```python
from build123d import *

# Parameters (mm, degrees)
SKETCH1_W                      = 27
SKETCH1_H                      = 35
SKETCH1_R                      = 1.113712744
SKETCH1_R_2                    = 1.000106258
SKETCH1_R_3                    = 1.174626552
SKETCH1_R_4                    = 1.19920455
SKETCH1_W_2                    = 8.5
SKETCH1_H_2                    = 2.12
BOSS_EXTRUDE1_DEPTH            = 2
SKETCH3_R                      = 2
BOSS_EXTRUDE2_DEPTH            = 2
M2_CLEARANCE_HOLE1_D           = 2.4
LPATTERN1_COUNT                = 2
LPATTERN1_PITCH                = 18
LPATTERN1_COUNT_DIR2           = 2
LPATTERN1_PITCH_DIR2           = 21.5
SKETCH6_W                      = 27
SKETCH6_H                      = 35
SKETCH6_W_2                    = 24
SKETCH6_H_2                    = 32
BOSS_EXTRUDE4_DEPTH            = 8.32
CUT_EXTRUDE1_REACH             = 41.261
SKETCH7_W                      = 8.5
SKETCH7_H                      = 5.57
CUT_EXTRUDE1_DIRECTION_2_DEPTH = 40.260756636
BOSS_EXTRUDE5_START            = -4
BOSS_EXTRUDE5_OUTLINE_R        = 1.2
BOSS_EXTRUDE5_DEPTH            = 2
M2_CLEARANCE_HOLE2_D           = 2.4
FILLET1_R                      = 2


with BuildPart() as part:
    # Sketch1 → Boss-Extrude1 (new body)
    # profile 1 of 8: a face of its own
    with BuildSketch(Plane(origin=(0, 0, 0), x_dir=(1, 0, 0), z_dir=(0, 1, 0))):
        with Locations((0.988085162, -0.939800033)):
            Rectangle(SKETCH1_W, SKETCH1_H)
        Polygon((-10.011914838, -15.939800033), (-10.011914838, 14.060199967), (11.988085162, 14.060199967), (11.988085162, -15.939800033), (5.238085162, -15.939800033), (5.238085162, -18.059800033), (-3.261914838, -18.059800033), (-3.261914838, -15.939800033), align=None, mode=Mode.SUBTRACT)
    # profile 2 of 8: a face of its own
    with BuildSketch(Plane(origin=(0, 0, 0), x_dir=(1, 0, 0), z_dir=(0, 1, 0))):
        Polygon((11.988085162, 14.060199967), (-10.011914838, 14.060199967), (-10.011914838, -15.939800033), (-3.261914838, -15.939800033), (-3.261914838, -13.819800033), (5.238085162, -13.819800033), (5.238085162, -15.939800033), (11.988085162, -15.939800033), align=None)
        with Locations((-8.011914838, -13.939800033)):
            Circle(SKETCH1_R, mode=Mode.SUBTRACT)
        with Locations((7.931487186, -14.291814947)):
            Circle(SKETCH1_R_2, mode=Mode.SUBTRACT)
        with Locations((-8.011914838, 7.560199967)):
            Circle(SKETCH1_R_3, mode=Mode.SUBTRACT)
        with Locations((9.988085162, 7.560199967)):
            Circle(SKETCH1_R_4, mode=Mode.SUBTRACT)
    # profile 3 of 8: a face of its own
    with BuildSketch(Plane(origin=(0, 0, 0), x_dir=(1, 0, 0), z_dir=(0, 1, 0))):
        with Locations((-8.011914838, 7.560199967)):
            Circle(SKETCH1_R_3)
    # profile 4 of 8: a face of its own
    with BuildSketch(Plane(origin=(0, 0, 0), x_dir=(1, 0, 0), z_dir=(0, 1, 0))):
        with Locations((9.988085162, 7.560199967)):
            Circle(SKETCH1_R_4)
    # profile 5 of 8: a face of its own
    with BuildSketch(Plane(origin=(0, 0, 0), x_dir=(1, 0, 0), z_dir=(0, 1, 0))):
        with Locations((7.931487186, -14.291814947)):
            Circle(SKETCH1_R_2)
    # profile 6 of 8: a face of its own
    with BuildSketch(Plane(origin=(0, 0, 0), x_dir=(1, 0, 0), z_dir=(0, 1, 0))):
        with Locations((0.988085162, -16.999800033)):
            Rectangle(SKETCH1_W_2, SKETCH1_H_2)
    # profile 7 of 8: a face of its own
    with BuildSketch(Plane(origin=(0, 0, 0), x_dir=(1, 0, 0), z_dir=(0, 1, 0))):
        with Locations((0.988085162, -14.879800033)):
            Rectangle(SKETCH1_W_2, SKETCH1_H_2)
    # profile 8 of 8: a face of its own
    with BuildSketch(Plane(origin=(0, 0, 0), x_dir=(1, 0, 0), z_dir=(0, 1, 0))):
        with Locations((-8.011914838, -13.939800033)):
            Circle(SKETCH1_R)
    extrude(amount=BOSS_EXTRUDE1_DEPTH)

    # Sketch3 → Boss-Extrude2 (add)
    with BuildSketch(Plane(origin=(0, 2, 0), x_dir=(1, 0, 0), z_dir=(0, 1, 0))):
        with Locations(Location((-8.011914838, 7.560199967, 0), (0, 0, 270))):
            Circle(SKETCH3_R)
    boss_extrude2 = extrude(amount=BOSS_EXTRUDE2_DEPTH)

    # M2 Clearance Hole1 (through all)
    with Locations(Plane(origin=(0, 4, 0), x_dir=(1, 0, 0), z_dir=(0, 1, 0))):
        with Locations((-8.011914838, 7.560199967)):
            m2_clearance_hole1 = Hole(M2_CLEARANCE_HOLE1_D / 2)

    # LPattern1: Boss-Extrude2, M2 Clearance Hole1 2 × 2
    with Locations(*[(i * LPATTERN1_PITCH, 0, j * LPATTERN1_PITCH_DIR2) for i in range(LPATTERN1_COUNT) for j in range(LPATTERN1_COUNT_DIR2) if (i, j) != (0, 0)]):
        add(boss_extrude2)
        add(m2_clearance_hole1, mode=Mode.SUBTRACT)

    # Sketch6 → Boss-Extrude4 (add)
    with BuildSketch(Plane(origin=(0, 2, 0), x_dir=(1, 0, 0), z_dir=(0, 1, 0))):
        with Locations((0.988085162, -0.939800033)):
            Rectangle(SKETCH6_W, SKETCH6_H)
        with Locations((0.988085162, -0.939800033)):
            Rectangle(SKETCH6_W_2, SKETCH6_H_2, mode=Mode.SUBTRACT)
    extrude(amount=BOSS_EXTRUDE4_DEPTH)

    # Sketch7 → Cut-Extrude1 (cut, up to next)
    with BuildSketch(Plane.XY.offset(18.439800033), mode=Mode.PRIVATE) as cut_extrude1_sk1:
        with Locations((0.988085162, 7.535)):
            Rectangle(SKETCH7_W, SKETCH7_H)
    cut_extrude1_tool1 = extrude(cut_extrude1_sk1.sketch, amount=-CUT_EXTRUDE1_REACH, mode=Mode.PRIVATE) & part.part
    add(cut_extrude1_tool1.solids().sort_by_distance((0.988085, 7.535, 18.4398))[0], mode=Mode.SUBTRACT)

    # Sketch7 → Cut-Extrude1 direction 2 (cut)
    with BuildSketch(Plane.XY.offset(18.439800033)):
        with Locations((0.988085162, 7.535)):
            Rectangle(SKETCH7_W, SKETCH7_H)
    extrude(amount=CUT_EXTRUDE1_DIRECTION_2_DEPTH, mode=Mode.SUBTRACT)

    # Boss-Extrude5: read off the stored shape, not the designer's step
    # Boss-Extrude5 outline → Boss-Extrude5 (add)
    with BuildSketch(Plane(origin=(0, 12.32, 0), x_dir=(1, 0, 0), z_dir=(0, 1, 0)).offset(BOSS_EXTRUDE5_START)):
        Polygon((-5.169409796, -23.439799853), (-5.169409796, -18.439799853), (-12.511914838, -18.439800033), (-12.511914838, 16.560199967), (14.488085162, 16.560199967), (14.488085162, -18.439800033), (7.002600417, -18.439800033), (7.002600417, -23.439799853), (19.488084722, -23.439799853), (19.488084722, 21.560200147), (-17.511915278, 21.560200147), (-17.511915278, -23.439799853), align=None)
        with Locations((-15.011915278, -20.939799853)):
            Circle(BOSS_EXTRUDE5_OUTLINE_R, mode=Mode.SUBTRACT)
        with Locations((16.988084722, -20.939799853)):
            Circle(BOSS_EXTRUDE5_OUTLINE_R, mode=Mode.SUBTRACT)
        with Locations((-15.011915278, 0)):
            Circle(BOSS_EXTRUDE5_OUTLINE_R, mode=Mode.SUBTRACT)
        with Locations((-15.011915278, 19.060200147)):
            Circle(BOSS_EXTRUDE5_OUTLINE_R, mode=Mode.SUBTRACT)
        with Locations((16.988084722, -0.939799853)):
            Circle(BOSS_EXTRUDE5_OUTLINE_R, mode=Mode.SUBTRACT)
        with Locations((16.988084722, 19.060200147)):
            Circle(BOSS_EXTRUDE5_OUTLINE_R, mode=Mode.SUBTRACT)
    extrude(amount=BOSS_EXTRUDE5_DEPTH)

    # M2 Clearance Hole2 (through all)
    with Locations(Plane(origin=(0, 10.32, 0), x_dir=(1, 0, 0), z_dir=(0, 1, 0))):
        with Locations((-15.011915278, 19.060200147), (-15.011915278, 0), (-15.011915278, -20.939799853), (16.988084722, -20.939799853), (16.988084722, -0.939799853), (16.988084722, 19.060200147)):
            Hole(M2_CLEARANCE_HOLE2_D / 2)

    # Fillet1
    # the kernel refuses this fillet: 2 mm, written as the material it adds along each edge
    with BuildSketch(Plane(origin=(7.002600417, 8.32, 18.439800033), x_dir=(0, 0, 1), z_dir=(0, 1, 0))) as fillet1_piece_1:
        with BuildLine():
            CenterArc((1.98608835, -2), FILLET1_R, 90, 83.23817367)
            Line((0, -1.764515255), (-0.039721767, -1.75980556))
            ThreePointArc((-0.039721767, -1.75980556), (-0.04, -0.882257627), (-0.04, 0))
            Line((-0.04, 0), (0, 0.04))
            Line((0, 0.04), (1.98608835, 0.04))
            Line((1.98608835, 0.04), (1.98608835, 0))
        make_face()
    extrude(amount=2)
    # the kernel refuses this fillet: 2 mm, written as the material it adds along each edge
    with BuildSketch(Plane(origin=(-5.169409796, 8.32, 18.439799853), x_dir=(0, 0, 1), z_dir=(0, 1, 0))) as fillet1_2_piece_1:
        with BuildLine():
            CenterArc((1.997859739, 2), FILLET1_R, 182.651020031, 87.348979969)
            Line((1.8e-07, 1.907494958), (-0.039957011, 1.905644857))
            ThreePointArc((-0.039957011, 1.905644857), (-0.03999982, 0.953747479), (-0.04, 0))
            Line((-0.04, 0), (0, -0.04))
            Line((0, -0.04), (1.997859739, -0.04))
            Line((1.997859739, -0.04), (1.997859739, 0))
        make_face()
    extrude(amount=2)
    # the kernel refuses this fillet: 2 mm, written as the material it takes off along each edge
    with BuildSketch(Plane(origin=(-5.169409796, 3.32, 23.439799853), x_dir=(0, 0, -1), z_dir=(0, 1, 0))) as fillet1_3_piece_1:
        with BuildLine():
            CenterArc((FILLET1_R, FILLET1_R), FILLET1_R, 180, 90)
            Line((0, FILLET1_R), (-FILLET1_R * 0.02, FILLET1_R))
            Line((-FILLET1_R * 0.02, FILLET1_R), (-FILLET1_R * 0.02, -FILLET1_R * 0.02))
            Line((-FILLET1_R * 0.02, -FILLET1_R * 0.02), (FILLET1_R, -FILLET1_R * 0.02))
            Line((FILLET1_R, -FILLET1_R * 0.02), (FILLET1_R, 0))
        make_face()
    extrude(amount=12, mode=Mode.SUBTRACT)
    # the kernel refuses this fillet: 2 mm, written as the material it takes off along each edge
    with BuildSketch(Plane(origin=(7.002600417, 3.32, 23.439799853), x_dir=(1, 0, 0), z_dir=(0, 1, 0))) as fillet1_4_piece_1:
        with BuildLine():
            CenterArc((FILLET1_R, FILLET1_R), FILLET1_R, 180, 90)
            Line((0, FILLET1_R), (-FILLET1_R * 0.02, FILLET1_R))
            Line((-FILLET1_R * 0.02, FILLET1_R), (-FILLET1_R * 0.02, -FILLET1_R * 0.02))
            Line((-FILLET1_R * 0.02, -FILLET1_R * 0.02), (FILLET1_R, -FILLET1_R * 0.02))
            Line((FILLET1_R, -FILLET1_R * 0.02), (FILLET1_R, 0))
        make_face()
    extrude(amount=12, mode=Mode.SUBTRACT)


solid = part.part
```
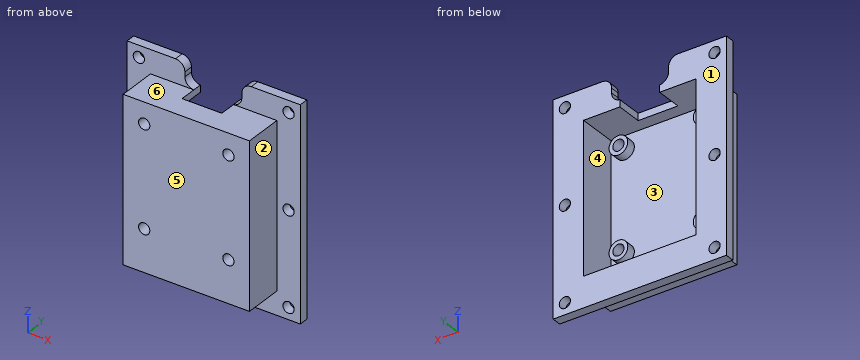
Check sheet for the modelled part. Datum: model origin and axes. Units: mm. Face numbers are marked on the shaded views. A direction names the side the tool comes from. Give positions to 0.01 mm unless a question says otherwise; leave off trailing zeros. Write each loop counter-clockwise with the first axis right and the second up, starting at its lowest first coordinate (ties: lowest second). Pieces come first, ordered by that corner, then holes. Notation, with made-up numbers: (10.25, 43) - (52.25, 43) arc R20 cw to (52.25, 47) - close; hole circle Ø8 at (19.5, 80). An arc over 180 degrees is marked (long way). Answer as a JSON object with one key per item and string values. Group by question number.
1) Depth check by flat-ended pin: P1, Ø4, axis at x = -8.01, z = 13.94, coming from the -Y side; P2, Ø4, axis at y = 2.5, z = -2, coming from the +X side; P3, Ø2, axis at y = 1.5, z = 5.5, coming from the -X side; P4, Ø3, axis at x = 16.99, z = 0.94, coming from the -Y side. Enter the tip coordinate at first touch or a pass-through.
2) Release check for a two-part mould opening along X. For the marked faces 1, 2 and 3 record: pulls with the +X half, pulls with the -X half, needs draft (parallel to the pull), parting line crosses it, or undercut.
3) Sectioned sample at C-C (y = 7). Record the cut outline in (x, z).
4) Access from +Z, -Z, +X, -X, +Y, -Y to the whole of each face (thin tool, end or side, straight path). Record for the marked faces 4, 5 and 6.
5) Sectioned sample at D-D (y = 9.5). Record the cut outline in (x, z), then the cut area to 3 significant figures.
6) Sectioned sample at A-A (y = 3.5). Give the number of separate pieces and of enclosed holes in the cut face, then the cut area to 3 significant figures.
7) Sectioned sample at B-B (x = 12.5). Record the cut outline in (y, z), then the cut area to 3 significant figures.
8) Thickness scan on probe 1 along X at (y, z) = (3, -7.5); probe 2 along X at (y, z) = (5.5, -4.5); probe 3 along X at (y, z) = (9.5, 12). Record the ranges inside material, lowest first. Write a range as from..to.
Geometry results:
{
 "1": {"P1": "stops at y = 0", "P2": "stops at x = 14.49", "P3": "stops at x = -12.51", "P4": "stops at y = 8.32"},
 "2": {"face 1": "needs draft", "face 2": "pulls with the +X half", "face 3": "undercut"},
 "3": {"outline": "(-12.51, -16.56) - (14.49, -16.56) - (14.49, 18.44) - (5.24, 18.44) - (5.24, 16.94) - (12.99, 16.94) - (12.99, -15.06) - (-11.01, -15.06) - (-11.01, 16.94) - (-3.26, 16.94) - (-3.26, 18.44) - (-12.51, 18.44) - close"},
 "4": {"face 4": "+Y", "face 5": "+Z, -Z, +X, -X, -Y", "face 6": "+Z, +X, -X, -Y"},
 "5": {"outline": "(-17.51, -21.56) - (19.49, -21.56) - (19.49, 23.44) - (9, 23.44) arc R2 ccw to (7, 21.44) - (7, 20.43) arc R2 cw to (5.24, 18.44) - (5.24, 16.94) - (12.99, 16.94) - (12.99, -15.06) - (-11.01, -15.06) - (-11.01, 16.94) - (-3.26, 16.94) - (-3.26, 18.44) arc R2 cw to (-5.17, 20.44) - (-5.17, 21.44) arc R2 ccw to (-7.17, 23.44) - (-17.51, 23.44) - close; hole circle Ø2.4 at (-15.01, -19.06); hole circle Ø2.4 at (-15.01, 0); hole circle Ø2.4 at (-15.01, 20.94); hole circle Ø2.4 at (16.99, -19.06); hole circle Ø2.4 at (16.99, 0.94); hole circle Ø2.4 at (16.99, 20.94)", "area": "796 mm^2"},
 "6": {"separate pieces": "5", "enclosed holes": "5", "area": "209 mm^2"},
 "7": {"outline": "(0, -16.56) - (8.32, -16.56) - (8.32, -21.56) - (10.32, -21.56) - (10.32, -15.06) - (2, -15.06) - (2, 16.94) - (10.32, 16.94) - (10.32, 23.44) - (8.32, 23.44) - (8.32, 18.44) - (0, 18.44) - close", "area": "115 mm^2"},
 "8": {"probe 1": "x = -12.51..-11.01, -10.01..-9.21, -6.81..-6.01, 7.99..8.79, 11.19..11.99, 12.99..14.49", "probe 2": "x = -12.51..-11.01, 12.99..14.49", "probe 3": "x = -17.51..-11.01, 12.99..19.49"}
}
